from build123d import *

# Parameters (mm, degrees)
SKETCH1_W            = 87
SKETCH1_H            = 50
BOSS_EXTRUDE1_DEPTH  = 2
SKETCH3_W            = 20
SKETCH3_H            = 6
BOSS_EXTRUDE2_DEPTH  = 5
CHAMFER1_SIZE        = 1.5
SKETCH4_W            = 10
SKETCH4_H            = 6
BOSS_EXTRUDE3_DEPTH  = 5
CHAMFER2_SIZE        = 1.5
SKETCH5_W            = 7
SKETCH5_H            = 2.5
BOSS_EXTRUDE4_DEPTH  = 6
M4_CLEARANCE_HOLE1_D = 4.5


with BuildPart() as part:
    # Sketch1 → Boss-Extrude1 (new body)
    with BuildSketch(Plane.XY):
        Rectangle(SKETCH1_W, SKETCH1_H)
    extrude(amount=BOSS_EXTRUDE1_DEPTH)

    # Sketch3 → Boss-Extrude2 (add)
    with BuildSketch(Plane(origin=(0, 25, 0), x_dir=(1, 0, 0), z_dir=(0, 1, 0))):
        with Locations((0, 3)):
            Rectangle(SKETCH3_W, SKETCH3_H)
    extrude(amount=-BOSS_EXTRUDE2_DEPTH)

    # Chamfer1
    chamfer1_edges = [part.edges().sort_by_distance(p)[0] for p in [
        (0, 20, -6),
        (0, 25, -6),
    ]]
    chamfer(chamfer1_edges, length=CHAMFER1_SIZE)

    # Sketch4 → Boss-Extrude3 (add)
    with BuildSketch(Plane.XZ.offset(25)):
        with Locations((-15, -3)):
            Rectangle(SKETCH4_W, SKETCH4_H)
    extrude(amount=-BOSS_EXTRUDE3_DEPTH)

    # Chamfer2
    chamfer2_edges = [part.edges().sort_by_distance(p)[0] for p in [
        (-15, -20, -6),
        (-15, -25, -6),
    ]]
    chamfer(chamfer2_edges, length=CHAMFER2_SIZE)

    # Sketch5 → Boss-Extrude4 (add)
    with BuildSketch(Plane(origin=(0, 0, 0), x_dir=(-1, 0, 0), z_dir=(0, 0, -1))):
        with Locations((-20, -23.75)):
            Rectangle(SKETCH5_W, SKETCH5_H)
    extrude(amount=BOSS_EXTRUDE4_DEPTH)

    # M4 Clearance Hole1 (through all)
    with Locations(Plane(origin=(0, 0, 0), x_dir=(-1, 0, 0), z_dir=(0, 0, -1))):
        with Locations((38.5, -20), (38.5, 20)):
            Hole(M4_CLEARANCE_HOLE1_D / 2)


solid = part.part
For this review, take the finished solid that the model builds, in its own axes (mm). A direction names the side the tool comes from. Round coordinates to 2 decimals unless told otherwise and drop trailing zeros. Loops run counter-clockwise (first coordinate to the right, second up) from the corner with the lowest first, then second, coordinate; pieces in that order, holes last. Notation, with made-up numbers: (85, 72) - (105, 72) arc R11 cw to (105, 80) - close; hole circle Ø8 at (62.5, -36.5). An arc over 180 degrees is marked (long way). Answer as CSV lines item,"result".
(1) Tool access review of faces 1 (the face through (-10, 23, -3)), 2 (the face through (-10, -23, -3)), 3 (the face through (23.5, -24, -3)): name each direction out of +Z, -Z, +X, -X, +Y, -Y from which nothing blocks a thin tool from reaching the whole face with its end or side.
Checked values:
face 1,"-Z, -X, +Y"
face 2,"-Z, -Y"
face 3,"-Z, +X, +Y, -Y"
(2) Consider section B-B on x = -38.5. Give the boundary of the cut face in (y, z), then the cut area to 3 significant figures.
Checked values:
outline,"(-25, 0) - (-22.25, 0) - (-22.25, 2) - (-25, 2) - close; (-17.75, 0) - (17.75, 0) - (17.75, 2) - (-17.75, 2) - close; (22.25, 0) - (25, 0) - (25, 2) - (22.25, 2) - close"
area,"82.0 mm2"
(3) Consider section D-D on y = 8. Give the boundary of the cut face in (x, z), then the cut area to 3 significant figures.
Checked values:
outline,"(-43.5, 0) - (43.5, 0) - (43.5, 2) - (-43.5, 2) - close"
area,"174 mm2"
(4) Consider section A-A on z = -3. Give the boundary of the cut face in (x, y), then the cut area to 4 significant figures.
Checked values:
outline,"(-20, -25) - (-10, -25) - (-10, -20) - (-20, -20) - close; (-10, 20) - (10, 20) - (10, 25) - (-10, 25) - close; (16.5, -25) - (23.5, -25) - (23.5, -22.5) - (16.5, -22.5) - close"
area,"167.5 mm2"
(5) Wall thickness on line 1 (Y direction, x = -38.5, z = 0.9); line 2 (Y direction, x = -8.5, z = -3.75); line 3 (Z direction, x = -37.5, y = -3.5): over which ranges is each line inside the solid? List them lowest first.
Checked values:
line 1,"y = -25 to -22.25, -17.75 to 17.75, 22.25 to 25"
line 2,"y = 20 to 25"
line 3,"z = 0 to 2"
(6) Insertion check: P1, Ø8, axis at x = -11.5, y = 5, coming from the -Z side; P2, Ø4, axis at x = -38.5, y = -20, coming from the -Z side (3 decimals); P3, Ø1.5, axis at y = 23.5, z = -2.5, coming from the -X side; P4, Ø1.3, axis at x = 5, z = -2, coming from the -Y side. Each pin has a flat end and moves straight along its axis. Give the tip position at first contact, or say it passes through.
Checked values:
P1,"stops at z = 0"
P2,"passes through"
P3,"stops at x = -10"
P4,"stops at y = 20"
(7) Mouldability with a two-part tool opening along Y and no side actions: class faces 4 (the face through (0, 20, -2)), 5 (the face through (-38.988, 17.804, 1.014)), 6 (the face through (10, 23, -3)) as +Y half, -Y half, draft (parallel to the pull), parting line (faces both ways), or undercut.
Checked values:
face 4,"-Y half"
face 5,"undercut"
face 6,"draft"
(8) Consider section C-C on x = 0.5. Give the boundary of the cut face in (y, z).
Checked values:
outline,"(-25, 0) - (20, 0) - (20, -4.5) - (21.5, -6) - (23.5, -6) - (25, -4.5) - (25, 2) - (-25, 2) - close"
